The model under review builds one solid part; all positions refer to its coordinate system, in mm. A direction names the side the tool comes from. Round coordinates to 2 decimals unless told otherwise and drop trailing zeros. Loops run counter-clockwise (first coordinate to the right, second up) from the corner with the lowest first, then second, coordinate; pieces in that order, holes last. Notation, with made-up numbers: (89, 20.25) -> (104, 20.25) arc R13 ccw to (104, 41.25) -> close; hole circle Ø7 at (65.25, -18.75). An arc over 180 degrees is marked (long way). Write each question's results on one line, items separated by ' | '. Start each with the question number.
Item 1: Mouldability with a two-part tool opening along Y and no side actions: class faces 1 (the flat face through (4, 3.55, -4)), 2 (the flat face through (0, 0, 0)), 3 (the flat face through (-4, 2.05, 0)) as pulls with the +Y half, pulls with the -Y half, needs draft (parallel to the pull), parting line crosses it, or undercut.
Item 2: Tool access review of faces 4 (the flat face through (2, 14.05, 3)), 5 (the cylindrical face through (4.336, 1.779, -19.524)), 6 (the cylindrical face through (-1.617, 7.374, -0.67)): name each direction out of +Z, -Z, +X, -X, +Y, -Y from which nothing blocks a thin tool from reaching the whole face with its end or side.
Item 3: We need section A-A (x = 0). Give the boundary of the cut face in (y, z), and give its area (3 significant figures).
Item 4: We need section B-B (y = 13.25). Give the boundary of the cut face in (x, z).
Item 5: For L1, parallel to Y at x = -12, z = -10; L2, parallel to Z at x = 0, y = 1.75; L3, parallel to Z at x = 0, y = 10.25, list the stretches that pass through material, from the lowest coordinate up. Write a range as from..to.
Item 6: Clearance check with flat-ended pins moving along their axes: pin 1 Ø6 at (y, z) = (2.5, -8.5) entering from -X; pin 2 Ø6 at (y, z) = (10, -4) entering from -X; pin 3 Ø5 at (x, y) = (1, 8.5) entering from -Z. State where each tip first meets the part, or that it passes through.
Item 7: We need section C-C (z = 0). Give the boundary of the cut face in (x, y).
from build123d import *

# Parameters (mm, degrees)
SKETCH1_W     = 2.25
SKETCH1_H     = 10.5
SKETCH1_W_2   = 20
SKETCH1_H_2   = 1.5
CHAMFER1_SIZE = 1.5
CHAMFER2_SIZE = 1


with BuildPart() as part:
    # Sketch1 → Revolve1 (revolve)
    with BuildSketch(Plane.XY):
        Polygon((-20, 3.55), (-20, 2.05), (-1.75, 2.05), (-1.75, 3.55), (-4, 3.55), align=None)
        Polygon((-22, 0), (-20, 0), (-20, 1.5), (-20, 2.05), (-20, 3.55), (-22, 3.55), align=None)
        with Locations((-2.875, 8.8)):
            Rectangle(SKETCH1_W, SKETCH1_H)
        with Locations((-10, 0.75)):
            Rectangle(SKETCH1_W_2, SKETCH1_H_2)
    revolve(axis=Axis((0, 0, 0), (0, 1, 0)))

    # Chamfer1
    chamfer1_edges = [part.edges().sort_by_distance(p)[0] for p in [
        (22, 0, 0),
        (22, 3.55, 0),
        (1.75, 14.05, 0),
    ]]
    chamfer(chamfer1_edges, length=CHAMFER1_SIZE)

    # Chamfer2
    chamfer2_edges = [part.edges().sort_by_distance(p)[0] for p in [
        (4, 3.55, 0),
    ]]
    chamfer(chamfer2_edges, length=CHAMFER2_SIZE)


solid = part.part
Here are the results:
1) face 1: pulls with the +Y half | face 2: pulls with the -Y half | face 3: undercut
2) face 4: +Z, -Z, +X, -X, +Y | face 5: none | face 6: +Y
3) outline: (0, -20.5) -> (1.5, -22) -> (2.05, -22) -> (3.55, -20.5) -> (3.55, -5) -> (4.55, -4) -> (14.05, -4) -> (14.05, -3.25) -> (12.55, -1.75) -> (2.05, -1.75) -> (2.05, -20) -> (1.5, -20) -> (1.5, 20) -> (2.05, 20) -> (2.05, 1.75) -> (12.55, 1.75) -> (14.05, 3.25) -> (14.05, 4) -> (4.55, 4) -> (3.55, 5) -> (3.55, 20.5) -> (2.05, 22) -> (1.5, 22) -> (0, 20.5) -> close | area: 170 mm2
4) outline: circle Ø8 at (0, 0); hole circle Ø4.9 at (0, 0)
5) L1: y = 0..1.5, 2.05..3.55 | L2: z = -22..-20, 20..22 | L3: z = -4..-1.75, 1.75..4
6) pin 1: stops at x = -21.29 | pin 2: stops at x = -3.87 | pin 3: stops at z = -4
7) outline: (-22, 1.5) -> (-20.5, 0) -> (20.5, 0) -> (22, 1.5) -> (22, 2.05) -> (20.5, 3.55) -> (5, 3.55) -> (4, 4.55) -> (4, 14.05) -> (3.25, 14.05) -> (1.75, 12.55) -> (1.75, 2.05) -> (20, 2.05) -> (20, 1.5) -> (-20, 1.5) -> (-20, 2.05) -> (-1.75, 2.05) -> (-1.75, 12.55) -> (-3.25, 14.05) -> (-4, 14.05) -> (-4, 4.55) -> (-5, 3.55) -> (-20.5, 3.55) -> (-22, 2.05) -> close
